Read the model definition and answer for the solid it produces. Units are mm, in the model's axes. Face numbers are marked on the shaded views. A direction names the side the tool comes from. Coordinates: 2 decimals unless noted, no trailing zeros. Loops run counter-clockwise (first coordinate to the right, second up) from the corner with the lowest first, then second, coordinate; pieces in that order, holes last.
Q1. Flat-ended cylindrical pins translate along their axes: P1, Ø11, axis at y = 381, z = 6, coming from the -X side; P2, Ø8, axis at x = 249, y = 323, coming from the +Z side; P3, Ø5, axis at x = 275.5, y = -61, coming from the -Z side; P4, Ø10, axis at x = 172, y = 480.5, coming from the -Z side. Find the tip coordinate at first contact, or state that the pin passes through.
Q2. Straight lines are drawn through the part: line 1 (Z direction, x = 282, y = 171.5); line 2 (Z direction, x = 274, y = 432.5); line 3 (Y direction, x = 180, z = 189). For each, find the intervals that lie inside material, in ascending order.
Q3. Section A-A (y = 162.5) is taken. Give the vertices of the cut face in (x, z), then the cut area to 3 significant figures.
Q4. Which of the six approach directions +Z, -Z, +X, -X, +Y, -Y give full straight-line access (tool end or side, diameter ignored) to the marked faces 3 and 4?
Q5. Section D-D (y = 510.5) is taken. Give the vertices of the cut face in (x, z), then the cut area to 3 significant figures.
Q6. Section B-B (x = 238) is taken. Give the vertices of the cut face in (y, z).
Q7. The mould has two halves that part along Y. Classify the marked faces 1 and 2: pulls with the +Y half, pulls with the -Y half, needs draft (parallel to the pull), parting line crosses it, or undercut.
Q8. Section C-C (z = 49.5) is taken. Give the vertices of the cut face in (x, y).
Solid Edge part; units mm, degrees
sketch "Sketch1" plane through (0, 0, 0) normal (0, 0, 1) x (1, 0, 0)
  circle A0 centre (230.5359, 171.3033) radius 50
  line L0 (180.0359, -178.6967) -> (281.0359, -178.6967)
  line L1 (281.0359, -178.6967) -> (281.0359, 521.3033)
  line L2 (281.0359, 521.3033) -> (180.0359, 521.3033)
  line L3 (180.0359, 521.3033) -> (180.0359, -178.6967)
  dimension "D1" = 180.0359
  dimension "D2" = 281.0359
extrude "Protrusion1" add sketch "Sketch1" along normal blind 10
sketch "Sketch2" plane through (-51.1743, -74.6061, 10) normal (0, 0, 1) x (0, 1, 0)
  circle A0 centre (585.9094, -281.7102) radius 60
  circle A1 centre (-94.0906, -281.7102) radius 60
extrude "ExtrudedProtrusion_3" add sketch "Sketch2" along normal blind 250
sketch "Sketch3" plane through (220.0359, 121.3033, 10) normal (0, 0, 1) x (0, -1, 0)
  circle A0 centre (-50, 10.5) radius 50
  circle A1 centre (-50, 10.5) radius 100
extrude "ExtrudedProtrusion_4" add sketch "Sketch3" against normal blind 20
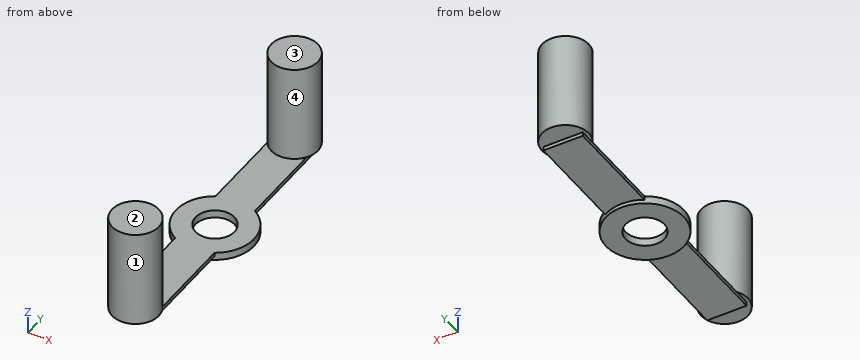
Numbers:
1. P1: stops at x = 180.04
1. P2: stops at z = 10
1. P3: stops at z = 0
1. P4: passes through
2. line 1: z = -10 to 10
2. line 2: z = 0 to 10
2. line 3: y = -201.04 to -136.35, 478.96 to 543.65
3. outline: (130.92, -10) - (181.32, -10) - (181.32, 10) - (130.92, 10) - close; (279.75, -10) - (330.15, -10) - (330.15, 10) - (279.75, 10) - close
3. area: 2,020 mm2
4. face 3: +Z, +X, -X, +Y, -Y
4. face 4: +Z
5. outline: (170.54, 10) - (180.04, 10) - (180.04, 0) - (281.04, 0) - (281.04, 10) - (290.53, 10) - (290.53, 260) - (170.54, 260) - close
5. area: 31,000 mm2
6. outline: (-228.23, 10) - (-178.7, 10) - (-178.7, 0) - (71.58, 0) - (71.58, -10) - (121.86, -10) - (121.86, 10) - (-109.16, 10) - (-109.16, 260) - (-228.23, 260) - close; (220.74, -10) - (271.02, -10) - (271.02, 0) - (521.3, 0) - (521.3, 10) - (570.84, 10) - (570.84, 260) - (451.77, 260) - (451.77, 10) - (220.74, 10) - close
7. face 1: undercut
7. face 2: needs draft
8. outline: circle Ø120 at (230.54, -168.7); circle Ø120 at (230.54, 511.3)
